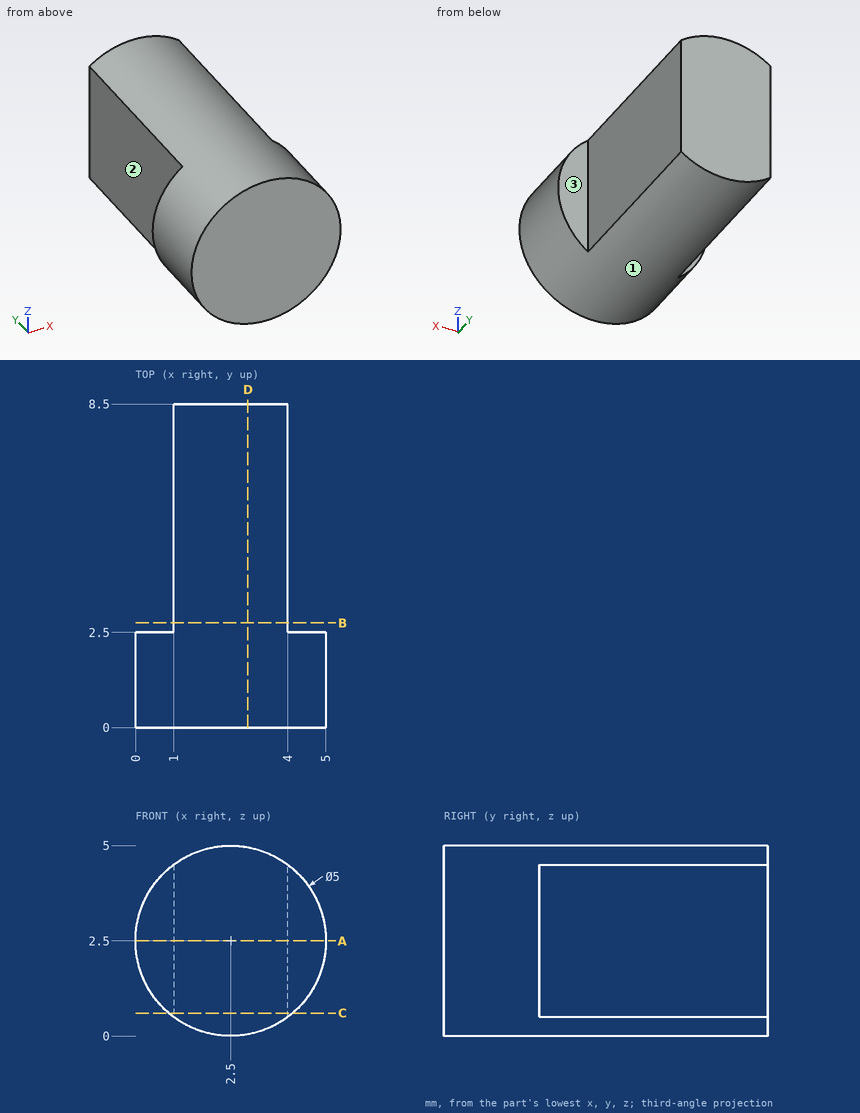
Verification items for this drawing (mm, ordinates from the low corner). A direction names the side the tool comes from. Give positions to 0.01 mm unless a question says otherwise; leave off trailing zeros. Write each loop counter-clockwise with the first axis right and the second up, starting at its lowest first coordinate (ties: lowest second). Pieces come first, ordered by that corner, then holes. Notation, with made-up numbers: (47.25, 44) -> (55.25, 44) arc R18 ccw to (55.25, 66) -> close; hole circle Ø1 at (73.5, 67). An arc over 180 degrees is marked (long way). Use CSV: the item, a comma, the result in double quotes. Start each with the question number.
Q1. Tool access check on the marked faces 1, 2 and 3. Record the directions out of +Z, -Z, +X, -X, +Y, -Y that give a thin tool (end or side, any length) a straight path to the whole face; none if there is none.
Q2. Cross-section at C-C on z = 0.6. Enter the section's corners in (x, y), and give its area (3 significant figures).
Q3. Cross-section at B-B on y = 2.75. Enter the section's corners in (x, z).
Q4. Scan lines: line 1 along X through (y, z) = (3.5, 3.7); line 2 along Z through (x, y) = (2.6, 4); line 3 along Y through (x, z) = (4.25, 3.75). Record each from-to range of solid material in increasing order.
Q5. Cross-section at A-A on z = 2.5. Enter the section's corners in (x, y), and give its area (3 significant figures).
Q6. Depth check by flat-ended pin: P1, Ø2, axis at x = 1.5, y = 1, coming from the -Z side; P2, Ø0.8, axis at x = 0.5, z = 3, coming from the +Y side; P3, Ø3, axis at y = 4.5, z = 3, coming from the +X side; P4, Ø1.2, axis at y = 5, z = 3.5, coming from the -X side. Enter the tip coordinate at first touch or a pass-through.
Q7. Cross-section at D-D on x = 2.95. Enter the section's corners in (y, z), and give its area (3 significant figures).
Working result:
1,face 1,"+Y, -Y"
1,face 2,"+Z, -Z, -X, +Y"
1,face 3,"+Z, -Z, +X, +Y"
2,outline,"(0.88, 0) -> (4.12, 0) -> (4.12, 2.5) -> (4, 2.5) -> (4, 8.5) -> (1, 8.5) -> (1, 2.5) -> (0.88, 2.5) -> close"
2,area,"26.1 mm^2"
3,outline,"(1, 0.5) arc R2.5 ccw to (4, 0.5) -> (4, 4.5) arc R2.5 ccw to (1, 4.5) -> close"
4,line 1,"x = 1 to 4"
4,line 2,"z = 0 to 5"
4,line 3,"y = 0 to 2.5"
5,outline,"(0, 0) -> (5, 0) -> (5, 2.5) -> (4, 2.5) -> (4, 8.5) -> (1, 8.5) -> (1, 2.5) -> (0, 2.5) -> close"
5,area,"30.5 mm^2"
6,P1,"stops at z = 0"
6,P2,"stops at y = 2.5"
6,P3,"stops at x = 4"
6,P4,"stops at x = 1"
7,outline,"(0, 0.04) -> (8.5, 0.04) -> (8.5, 4.96) -> (0, 4.96) -> close"
7,area,"41.8 mm^2"
